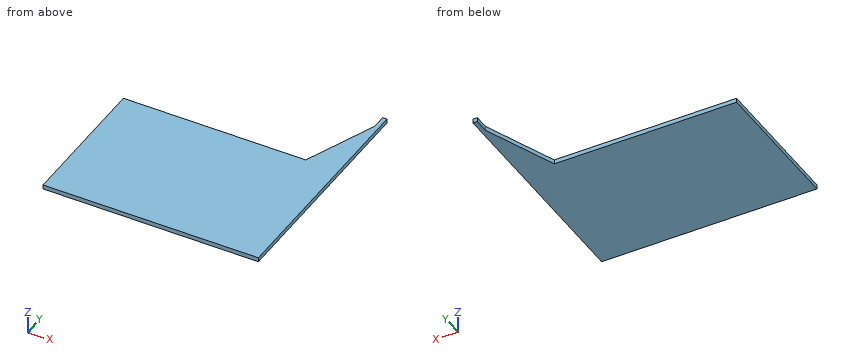
Autodesk Inventor part; units mm, degrees
ref_plane "YZ Plane" through (0, 0, 0) normal (1, 0, 0) x (0, 1, 0)
ref_plane "XZ Plane" through (0, 0, 0) normal (0, 1, 0) x (-1, 0, 0)
ref_plane "XY Plane" through (0, 0, 0) normal (0, 0, 1) x (1, 0, 0)
sketch "Boceto1" plane through (0, 0, 0) normal (0, 0, 1) x (1, 0, 0)
  line L0 (0, 0) -> (150, 0)
  line L1 (150, 0) -> (150, 100)
  line L2 (150, 100) -> (0, 100)
  line L3 (0, 100) -> (0, 0)
  dimension "d0" = 150
  dimension "d1" = 100
extrude "Extrusión1" add sketch "Boceto1" along normal blind 3
sketch "Boceto2" plane through (0, 100, 0) normal (0, 1, 0) x (1, 0, 0)
  line L0 (150, 0) -> (0, 0) construction
  line L1 (0, 0) -> (0, -3) construction
  line L2 (150, -3) -> (0, -3) construction
  line L3 (150, 0) -> (150, -3) construction
  line L4 (150, 0) -> (147, 0)
  line L5 (147, 0) -> (147, -3)
  line L6 (147, -3) -> (150, -3)
  line L7 (150, -3) -> (150, 0)
  line L8 (150, 0) -> (150, -3) construction
  line L9 (150, -3) -> (0, -3) construction
  point P0 (0, 0)
  dimension "d4" = 3
  dimension "d5" = 3
extrude "Extrusión2" add sketch "Boceto2" along normal blind 60
sketch "Boceto3" plane through (0, 0, 3) normal (0, 0, 1) x (1, 0, 0)
  line L0 (0, 0) -> (150, 0) construction
  line L1 (150, 0) -> (150, 160) construction
  line L2 (147, 160) -> (150, 160) construction
  line L3 (147, 100) -> (147, 160) construction
  line L4 (147, 100) -> (0, 100) construction
  line L5 (0, 100) -> (0, 0) construction
  line L6 (147, 100) -> (127, 100)
  line L7 (147, 100) -> (0, 100) construction
  line L8 (127, 100) -> (147, 150)
  line L9 (147, 100) -> (147, 160) construction
  line L10 (147, 150) -> (147, 100)
  dimension "d8" = 20
  dimension "d9" = 10
extrude "Extrusión3" add sketch "Boceto3" against normal blind 3
properties part number "Porton"
Verification items for the finished model (mm, model axes). Give positions to 0.01 mm unless a question says otherwise; leave off trailing zeros. Write each loop counter-clockwise with the first axis right and the second up, starting at its lowest first coordinate (ties: lowest second). Pieces come first, ordered by that corner, then holes. Notation, with made-up numbers: (-26.5, 82.25) -> (19.5, 82.25) arc R29 ccw to (19.5, 112.25) -> close; hole circle Ø3 at (71, -18.5). An arc over 180 degrees is marked (long way). Use CSV: the item, a comma, the result in double quotes.
(1) Sectioned sample at B-B (x = 25). Record the cut outline in (y, z), plus the area to 3 significant figures.
Derived:
outline,"(0, 0) -> (100, 0) -> (100, 3) -> (0, 3) -> close"
area,"300 mm^2"
(2) Go/stop test with a flat-tipped pin: pin 1 (1.5 mm diameter, centred on x = 71, z = 1.5, fed in from +Y). Record where the tip stops, or that it passes through.
Derived:
pin 1,"stops at y = 100"
(3) Sectioned sample at A-A (z = 2.15). Record the cut outline in (x, y).
Derived:
outline,"(0, 0) -> (150, 0) -> (150, 160) -> (147, 160) -> (147, 150) -> (127, 100) -> (0, 100) -> close"
(4) Material ranges on L1, parallel to Y at x = 81, z = 1.5; L2, parallel to X at y = 152, z = 0.45; L3, parallel to X at y = 121, z = 0.45, recorded low to high.
Derived:
L1,"y = 0 to 100"
L2,"x = 147 to 150"
L3,"x = 135.4 to 150"
(5) Sectioned sample at C-C (y = 108). Record the cut outline in (x, z).
Derived:
outline,"(130.2, 0) -> (150, 0) -> (150, 3) -> (130.2, 3) -> close"
